Geometry: see drawing. Coordinates: mm, zero at the bounding-box minimum. A direction names the side the tool comes from. Round coordinates to 2 decimals unless told otherwise and drop trailing zeros. Loops run counter-clockwise (first coordinate to the right, second up) from the corner with the lowest first, then second, coordinate; pieces in that order, holes last. Notation, with made-up numbers: (10, 1) - (36, 1) arc R11 ccw to (36, 13) - close; hole circle Ø5 at (-13, 22.5). An arc over 180 degrees is marked (long way). Use CSV: the item, a comma, the result in double quotes.
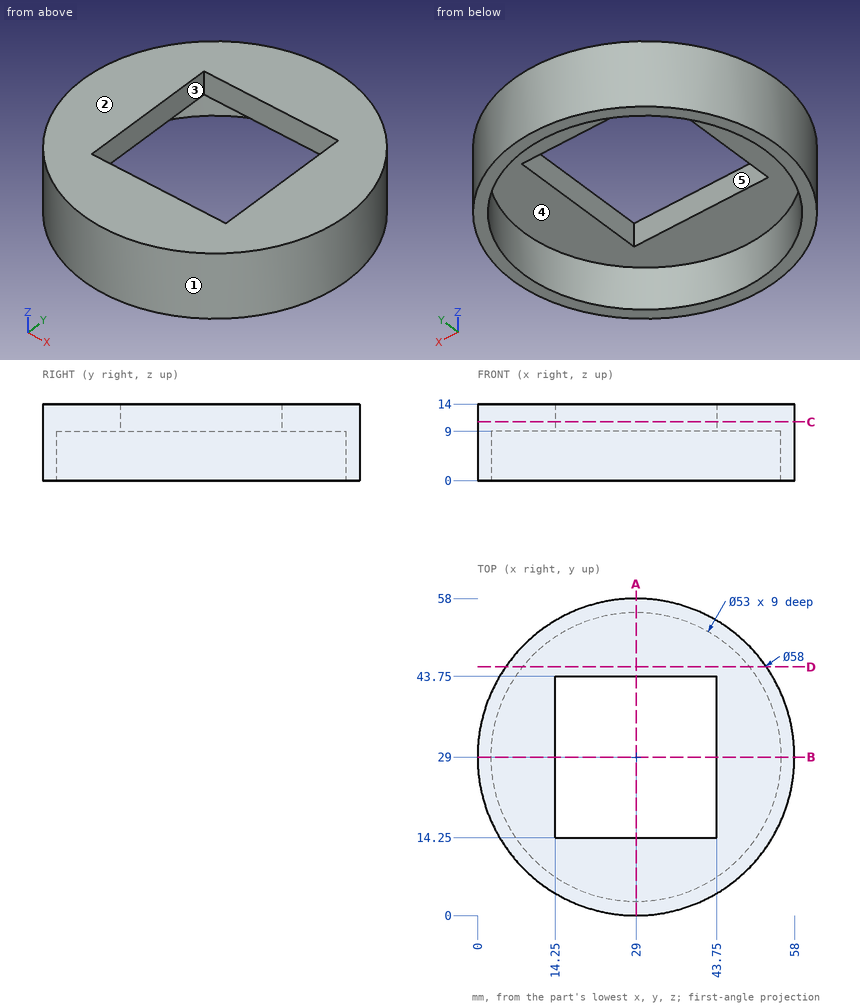
Item 1: Pin query (flat end, axial travel): P1, Ø5, axis at y = 38, z = 9, coming from the -X side; P2, Ø5, axis at y = 41, z = 12.5, coming from the -X side; P3, Ø4, axis at x = 31, z = 12, coming from the +Y side. Return the tip coordinate at first contact, or that it passes through.
Final values:
P1,"stops at x = 0.74"
P2,"stops at x = 1.6"
P3,"stops at y = 58"
Item 2: Reachability of the marked faces 4 and 5 from +Z, -Z, +X, -X, +Y, -Y: full face, straight path, thin tool, end or side. Return the list, or none.
Final values:
face 4,"-Z"
face 5,"+Z, -Z"
Item 3: Section C-C on z = 10.75. Return the cut outline in (x, y).
Final values:
outline,"circle Ø58 at (29, 29); hole (14.25, 14.25) - (43.75, 14.25) - (43.75, 43.75) - (14.25, 43.75) - close"
Item 4: Section D-D on y = 45.5. Return the cut outline in (x, z).
Final values:
outline,"(5.15, 0) - (8.26, 0) - (8.26, 9) - (49.74, 9) - (49.74, 0) - (52.85, 0) - (52.85, 14) - (5.15, 14) - close"
Item 5: Material intervals for line 1 (Y direction, x = 29, z = 6.5); line 2 (Y direction, x = 9.5, z = 3.5); line 3 (X direction, y = 5, z = 8), sorted ascending.
Final values:
line 1,"y = 0 to 2.5, 55.5 to 58"
line 2,"y = 7.53 to 11.06, 46.94 to 50.47"
line 3,"x = 12.72 to 17.76, 40.24 to 45.28"
Item 6: Mould query, pull axis X, two halves, no side actions, for the marked faces 1, 2 and 3. Classes: released by +X, released by -X, zero draft, split by the parting line, or undercut.
Final values:
face 1,"split by the parting line"
face 2,"zero draft"
face 3,"undercut"
Item 7: Section A-A on x = 29. Return the cut outline in (y, z).
Final values:
outline,"(0, 0) - (2.5, 0) - (2.5, 9) - (14.25, 9) - (14.25, 14) - (0, 14) - close; (43.75, 9) - (55.5, 9) - (55.5, 0) - (58, 0) - (58, 14) - (43.75, 14) - close"
